Input: part model. Units: mm. Frame: model coordinates. Coordinates: 2 decimals unless noted, no trailing zeros. Order: outer loops, then holes, each group sorted by start corner. A loop starts at its lowest first (then second) coordinate and runs counter-clockwise, first axis right, second up. Notation, with made-up numbers: (70, 63.5) -> (119, 63.5) arc R26 ccw to (119, 85.5) -> close; hole circle Ø7 at (32.5, -26). An arc over 180 degrees is marked (long way). Answer as CSV lines item,"result".
from build123d import *

# Parameters (mm, degrees)
SKETCH1_R           = 3.175
BOSS_EXTRUDE1_DEPTH = 6.35


with BuildPart() as part:
    # Sketch1 → Boss-Extrude1 (new body)
    with BuildSketch(Plane.XY):
        Polygon((-82.55, 12.7), (-76.2, 12.7), (-76.2, 6.35), (-69.85, 6.35), (-69.85, 12.7), (-63.5, 12.7), (-63.5, 6.35), (-57.15, 6.35), (-57.15, 12.7), (-50.8, 12.7), (-50.8, 6.35), (-44.45, 6.35), (-44.45, 12.7), (-38.1, 12.7), (-38.1, 6.35), (-31.75, 6.35), (-31.75, 12.7), (-25.4, 12.7), (-25.4, 6.35), (-19.05, 6.35), (-19.05, 12.7), (-12.7, 12.7), (-12.7, 6.35), (-6.35, 6.35), (-6.35, 12.7), (6.35, 12.7), (6.35, 6.35), (12.7, 6.35), (12.7, 12.7), (19.05, 12.7), (19.05, 6.35), (25.4, 6.35), (25.4, 12.7), (31.75, 12.7), (31.75, 6.35), (38.1, 6.35), (38.1, 12.7), (44.45, 12.7), (44.45, 6.35), (50.8, 6.35), (50.8, 12.7), (57.15, 12.7), (57.15, 6.35), (63.5, 6.35), (63.5, 12.7), (69.85, 12.7), (69.85, 6.35), (76.2, 6.35), (76.2, 12.7), (82.55, 12.7), (82.55, 6.35), (95.167491893, 6.35), (95.167491893, -6.35), (82.55, -6.35), (82.55, -12.7), (76.2, -12.7), (76.2, -6.35), (69.85, -6.35), (69.85, -12.7), (63.5, -12.7), (63.5, -6.35), (57.15, -6.35), (57.15, -12.7), (50.8, -12.7), (50.8, -6.35), (44.45, -6.35), (44.45, -12.7), (38.1, -12.7), (38.1, -6.35), (31.75, -6.35), (31.75, -12.7), (25.4, -12.7), (25.4, -6.35), (19.05, -6.35), (19.05, -12.7), (12.7, -12.7), (12.7, -6.35), (6.35, -6.35), (6.35, -12.7), (-6.35, -12.7), (-6.35, -6.35), (-12.7, -6.35), (-12.7, -12.7), (-19.05, -12.7), (-19.05, -6.35), (-25.4, -6.35), (-25.4, -12.7), (-31.75, -12.7), (-31.75, -6.35), (-38.1, -6.35), (-38.1, -12.7), (-44.45, -12.7), (-44.45, -6.35), (-50.8, -6.35), (-50.8, -12.7), (-57.15, -12.7), (-57.15, -6.35), (-63.5, -6.35), (-63.5, -12.7), (-69.85, -12.7), (-69.85, -6.35), (-76.2, -6.35), (-76.2, -12.7), (-82.55, -12.7), (-82.55, -6.35), (-95.167491893, -6.35), (-95.167491893, 6.35), (-82.55, 6.35), align=None)
        with Locations((79.292491893, 0)):
            Circle(SKETCH1_R, mode=Mode.SUBTRACT)
        with Locations((53.892491893, 0)):
            Circle(SKETCH1_R, mode=Mode.SUBTRACT)
    extrude(amount=BOSS_EXTRUDE1_DEPTH)


solid = part.part
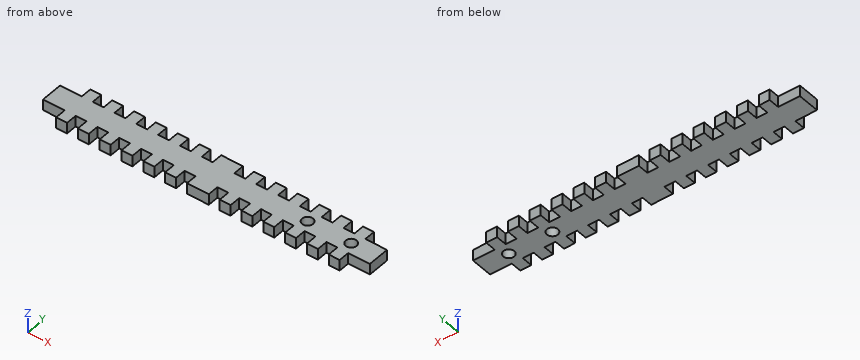
1. Ray query, line 1 along X through (y, z) = (-2.25, 4); line 2 along X through (y, z) = (-2, 2); line 3 along Y through (x, z) = (-84.5, 2.25). Return the intervals inside material, ascending.
Findings:
line 1,"x = -95.17 to 51.65, 56.13 to 77.05, 81.53 to 95.17"
line 2,"x = -95.17 to 51.43, 56.36 to 76.83, 81.76 to 95.17"
line 3,"y = -6.35 to 6.35"
2. Cut plane A-A (y = 0). Return the cut outline in (x, z).
Findings:
outline,"(-95.17, 0) -> (50.72, 0) -> (50.72, 6.35) -> (-95.17, 6.35) -> close; (57.07, 0) -> (76.12, 0) -> (76.12, 6.35) -> (57.07, 6.35) -> close; (82.47, 0) -> (95.17, 0) -> (95.17, 6.35) -> (82.47, 6.35) -> close"
3. Cut plane C-C (x = -72.5). Return the cut outline in (y, z), plus the area to 3 significant figures.
Findings:
outline,"(-6.35, 0) -> (6.35, 0) -> (6.35, 6.35) -> (-6.35, 6.35) -> close"
area,"80.6 mm2"
4. Contact query for flat-ended pins moving along their axis: pin 1 (3 mm diameter, centred on x = -22.5, z = 5.5, fed in from +Y); pin 2 (6 mm diameter, centred on x = -10.5, y = -9, fed in from -Z); pin 3 (1.9 mm diameter, centred on y = -10, z = 1.5, fed in from -X); pin 4 (3 mm diameter, centred on x = -73, z = 4.5, fed in from -Y). Output: stop coordinate, or through.
Findings:
pin 1,"stops at y = 6.35"
pin 2,"stops at z = 0"
pin 3,"stops at x = -82.55"
pin 4,"stops at y = -6.35"
5. Cut plane B-B (z = 3). State how many separate pieces and enclosed holes the cut face has, plus the area to 3 significant figures.
Findings:
separate pieces,"1"
enclosed holes,"2"
area,"3,480 mm2"
